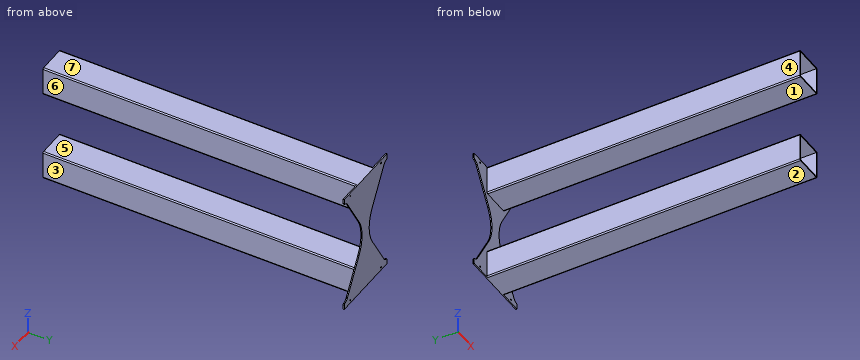
from build123d import *

# Parameters (mm, degrees)
SKETCH1_R           = 1.5875
BOSS_EXTRUDE1_DEPTH = 2.54
SKETCH2_W           = 63.5
SKETCH2_H           = 63.5
BOSS_EXTRUDE2_DEPTH = 685.8
SHELL1_START        = -688.34
SHELL1_OUTLINE_W    = 58.42
SHELL1_OUTLINE_H    = 58.42
SHELL1_DEPTH        = 685.8
FILLET1_R           = 2.54
FILLET2_R           = 2.54


# Read off the part's stored shape, not the designer's step: Shell1
with BuildPart() as part:
    # Sketch1 → Boss-Extrude1 (new body)
    with BuildSketch(Plane(origin=(0, 0, 0), x_dir=(1, 0, 0), z_dir=(0, 1, 0))):
        with BuildLine():
            Line((-79.375, -133.985), (79.375, -133.985))
            Line((79.375, -133.985), (79.375, -123.618732018))
            ThreePointArc((79.375, -123.618732018), (78.770533054, -121.973948811), (77.244833229, -121.1120137))
            ThreePointArc((77.244833229, -121.1120137), (71.931312021, -118.98641106), (68.016545719, -114.811929173))
            Line((68.016545719, -114.811929173), (24.542448632, -41.427653291))
            ThreePointArc((24.542448632, -41.427653291), (13.192327388, 0), (24.542448632, 41.427653291))
            Line((24.542448632, 41.427653291), (68.016545719, 114.811929173))
            ThreePointArc((68.016545719, 114.811929173), (71.931312021, 118.98641106), (77.244833229, 121.1120137))
            ThreePointArc((77.244833229, 121.1120137), (78.770533054, 121.973948811), (79.375, 123.618732018))
            Line((79.375, 123.618732018), (79.375, 133.985))
            Line((79.375, 133.985), (-79.375, 133.985))
            Line((-79.375, 133.985), (-79.375, 123.618732018))
            ThreePointArc((-79.375, 123.618732018), (-78.770533054, 121.973948811), (-77.244833229, 121.1120137))
            ThreePointArc((-77.244833229, 121.1120137), (-71.931312021, 118.98641106), (-68.016545719, 114.811929173))
            Line((-68.016545719, 114.811929173), (-24.542448632, 41.427653291))
            ThreePointArc((-24.542448632, 41.427653291), (-13.192327388, 0), (-24.542448632, -41.427653291))
            Line((-24.542448632, -41.427653291), (-68.016545719, -114.811929173))
            ThreePointArc((-68.016545719, -114.811929173), (-71.931312021, -118.98641106), (-77.244833229, -121.1120137))
            ThreePointArc((-77.244833229, -121.1120137), (-78.770533054, -121.973948811), (-79.375, -123.618732018))
            Line((-79.375, -123.618732018), (-79.375, -133.985))
        make_face()
        with Locations(Location((-57.15, 127, 0), (0, 0, 270))):
            Circle(SKETCH1_R, mode=Mode.SUBTRACT)
        with Locations(Location((57.15, 127, 0), (0, 0, 270))):
            Circle(SKETCH1_R, mode=Mode.SUBTRACT)
        with Locations(Location((57.15, -127, 0), (0, 0, 90))):
            Circle(SKETCH1_R, mode=Mode.SUBTRACT)
        with Locations(Location((-57.15, -127, 0), (0, 0, 90))):
            Circle(SKETCH1_R, mode=Mode.SUBTRACT)
    extrude(amount=-BOSS_EXTRUDE1_DEPTH)

    # Sketch2 → Boss-Extrude2 (add)
    with BuildSketch(Plane.XZ.offset(2.54)):
        with Locations((0, -102.235)):
            Rectangle(SKETCH2_W, SKETCH2_H)
        with Locations((0, 102.235)):
            Rectangle(SKETCH2_W, SKETCH2_H)
    extrude(amount=BOSS_EXTRUDE2_DEPTH)

    # Shell1 outline → Shell1 (cut)
    with BuildSketch(Plane(origin=(0, 0, 0), x_dir=(1, 0, 0), z_dir=(0, 1, 0)).offset(SHELL1_START)):
        with Locations((0, 102.235)):
            Rectangle(SHELL1_OUTLINE_W, SHELL1_OUTLINE_H)
        with Locations((0, -102.235)):
            Rectangle(SHELL1_OUTLINE_W, SHELL1_OUTLINE_H)
    extrude(amount=SHELL1_DEPTH, mode=Mode.SUBTRACT)

    # Fillet1
    fillet1_edges = [part.edges().sort_by_distance(p)[0] for p in [
        (31.75, -345.44, 70.485),
        (31.75, -345.44, 133.985),
        (-31.75, -345.44, 133.985),
        (-31.75, -345.44, 70.485),
    ]]
    fillet(fillet1_edges, radius=FILLET1_R)

    # Fillet2
    fillet2_edges = [part.edges().sort_by_distance(p)[0] for p in [
        (-31.75, -345.44, -70.485),
        (-31.75, -345.44, -133.985),
        (31.75, -345.44, -133.985),
        (31.75, -345.44, -70.485),
    ]]
    fillet(fillet2_edges, radius=FILLET2_R)


solid = part.part
Work out the finished part from the listing and answer in its coordinate system (mm). Face numbers are marked on the shaded views. A direction names the side the tool comes from. Give positions to 0.01 mm unless a question says otherwise; leave off trailing zeros. Loops run counter-clockwise (first coordinate to the right, second up) from the corner with the lowest first, then second, coordinate; pieces in that order, holes last. Notation, with made-up numbers: (4.5, -12) - (14.5, -12) arc R16 cw to (14.5, -5) - close; hole circle Ø7 at (19, 17). An arc over 180 degrees is marked (long way). Answer in a Markdown table with one row per item. Add a question column.
Q1. The part is cut by section A-A (y = -79). Determine the outline of the cut face in (x, z) (3 decimals).
Q2. Consider line 1 along Z through (x, y) = (19.5, -377.5) (3 decimals); line 2 along X through (y, z) = (-0.6, -127) (1 decimal); line 3 along X through (y, z) = (-574, -122). Determine where each line is inside the solid, lowest interval first.
Q3. A tool of negligible diameter and unlimited length cuts with its end or side. For the marked faces 4, 5, 6 and 7, from which of +Z, -Z, +X, -X, +Y, -Y can it reach the whole face along a straight path? Write none if from no direction.
Q4. Determine the mould class of the marked faces 1, 2 and 3 for opening direction Z: released by +Z, released by -Z, zero draft, split by the parting line, or undercut.
Q5. The part is cut by section C-C (x = 41). Determine the outline of the cut face in (y, z) (3 decimals), and give its area (3 significant figures).
Q6. Each of these flat-tipped pins is pushed along its axis until it touches: P1, Ø17.5, axis at y = -218.5, z = -112.5, coming from the -X side; P2, Ø6, axis at x = 60, z = -93.5, coming from the +Y side; P3, Ø4, axis at y = -454.5, z = -94, coming from the +X side. Where does it stop, or does it pass through?
Q7. The part is cut by section D-D (z = -17.5). Determine the outline of the cut face in (x, y).
Q8. The part is cut by section B-B (x = -4). Determine the outline of the cut face in (y, z) (3 decimals).
Solution:
| question | item | result |
|---|---|---|
| 1 | outline | (-31.75, -131.445) arc R2.54 ccw to (-29.21, -133.985) - (29.21, -133.985) arc R2.54 ccw to (31.75, -131.445) - (31.75, -73.025) arc R2.54 ccw to (29.21, -70.485) - (-29.21, -70.485) arc R2.54 ccw to (-31.75, -73.025) - close; (-31.75, 73.025) arc R2.54 ccw to (-29.21, 70.485) - (29.21, 70.485) arc R2.54 ccw to (31.75, 73.025) - (31.75, 131.445) arc R2.54 ccw to (29.21, 133.985) - (-29.21, 133.985) arc R2.54 ccw to (-31.75, 131.445) - close; hole (-29.21, -131.445) - (29.21, -131.445) - (29.21, -73.025) - (-29.21, -73.025) - close; hole (-29.21, 73.025) - (29.21, 73.025) - (29.21, 131.445) - (-29.21, 131.445) - close |
| 2 | line 1 | z = -133.985 to -131.445, -73.025 to -70.485, 70.485 to 73.025, 131.445 to 133.985 |
| 2 | line 2 | x = -79.4 to -58.7, -55.6 to 55.6, 58.7 to 79.4 |
| 2 | line 3 | x = -31.75 to -29.21, 29.21 to 31.75 |
| 3 | face 4 | +Z, -Z, -X, -Y |
| 3 | face 5 | +X, -X, -Y |
| 3 | face 6 | +Z, -Z, +X, -Y |
| 3 | face 7 | +Z, +X, -X, +Y, -Y |
| 4 | face 1 | undercut |
| 4 | face 2 | released by -Z |
| 4 | face 3 | zero draft |
| 5 | outline | (-2.54, -133.985) - (0, -133.985) - (0, -69.208) - (-2.54, -69.208) - close; (-2.54, 69.208) - (0, 69.208) - (0, 133.985) - (-2.54, 133.985) - close |
| 5 | area | 329 mm² |
| 6 | P1 | stops at x = -31.75 |
| 6 | P2 | passes through |
| 6 | P3 | stops at x = 31.75 |
| 7 | outline | (-15.1, -2.54) - (15.1, -2.54) - (15.1, 0) - (-15.1, 0) - close |
| 8 | outline | (-688.34, -133.985) - (0, -133.985) - (0, 133.985) - (-688.34, 133.985) - (-688.34, 131.445) - (-2.54, 131.445) - (-2.54, 73.025) - (-688.34, 73.025) - (-688.34, 70.485) - (-2.54, 70.485) - (-2.54, -70.485) - (-688.34, -70.485) - (-688.34, -73.025) - (-2.54, -73.025) - (-2.54, -131.445) - (-688.34, -131.445) - close |
